Verification items for the finished model (mm, model axes). Round coordinates to 2 decimals unless told otherwise and drop trailing zeros. Order: outer loops, then holes, each group sorted by start corner. A loop starts at its lowest first (then second) coordinate and runs counter-clockwise, first axis right, second up. Notation, with made-up numbers: (80.25, 7.25) -> (119.25, 7.25) arc R28 ccw to (119.25, 45.25) -> close; hole circle Ø8 at (-28, 48). An arc over 180 degrees is marked (long way). Put each result on its own line as item: value.
Autodesk Inventor part; units mm, degrees
ref_plane "YZ Plane" through (0, 0, 0) normal (1, 0, 0) x (0, 1, 0)
ref_plane "XZ Plane" through (0, 0, 0) normal (0, 1, 0) x (-1, 0, 0)
ref_plane "XY Plane" through (0, 0, 0) normal (0, 0, 1) x (1, 0, 0)
sketch "スケッチ1" plane through (0, 0, 0) normal (0, 0, 1) x (1, 0, 0)
  line L0 (0, 0) -> (45, 0)
  line L1 (45, 0) -> (45, 100)
  line L2 (45, 100) -> (0, 100)
  line L3 (0, 100) -> (0, 0)
  dimension "d0" = 100
  dimension "d1" = 45
extrude "押し出し1" add sketch "スケッチ1" along normal blind 5
sketch "スケッチ2" plane through (0, 0, 5) normal (0, 0, 1) x (1, 0, 0)
  line L0 (0, 0) -> (45, 0)
  point P0 (22.6447, 79.5)
  dimension "d4" = 79.5
hole "穴1" at (22.6447, 79.5, 5) direction (0, 0, -1) diameter 24 end through all
sketch "スケッチ3" plane through (0, 0, 0) normal (0, 0, -1) x (-1, 0, 0)
  line L0 (0, 0) -> (-45, 0)
  line L1 (-45, 0) -> (-45, 100)
  line L2 (0, 100) -> (0, 0)
  point P0 (-10, 10)
  point P1 (-35, 10)
  dimension "d12" = 10
  dimension "d13" = 10
  dimension "d14" = 10
  dimension "d15" = 10
hole "穴2" at (10, 10, 0) at (35, 10, 0) direction (0, 0, 1) diameter 5 end through all
sketch "スケッチ4" plane through (0, 0, 5) normal (0, 0, 1) x (1, 0, 0)
  line L0 (0, 100) -> (0, 0)
  line L1 (0, 0) -> (45, 0)
  point P0 (22.5, 30)
  dimension "d23" = 22.5
  dimension "d24" = 30
hole "穴3" at (22.5, 30, 5) direction (0, 0, -1) diameter 15 depth 8 tip angle 118
properties part number "回転軸取り付け板"
Item 1: Sectioned sample at A-A, the plane y = 10. Record the boundary of the cut face in (x, z), then the cut area to 3 significant figures.
Geometry check:
outline: (0, 0) -> (7.5, 0) -> (7.5, 5) -> (0, 5) -> close; (12.5, 0) -> (32.5, 0) -> (32.5, 5) -> (12.5, 5) -> close; (37.5, 0) -> (45, 0) -> (45, 5) -> (37.5, 5) -> close
area: 175 mm2
Item 2: Release check for a two-part mould opening along Y. For faces 1 (the face through (22, 0, 2)), 2 (the face through (12.44, 9.46, 2.54)), 3 (the face through (22, 51, 0)) record: pulls with the +Y half, pulls with the -Y half, needs draft (parallel to the pull), parting line crosses it, or undercut.
Geometry check:
face 1: pulls with the -Y half
face 2: undercut
face 3: needs draft
Item 3: Sectioned sample at C-C, the plane z = 3. Record the boundary of the cut face in (x, y).
Geometry check:
outline: (0, 0) -> (45, 0) -> (45, 100) -> (0, 100) -> close; hole circle Ø5 at (10, 10); hole circle Ø24 at (22.64, 79.5); hole circle Ø15 at (22.5, 30); hole circle Ø5 at (35, 10)
Item 4: Sectioned sample at D-D, the plane y = 35. Record the boundary of the cut face in (x, z), then the cut area to 3 significant figures.
Geometry check:
outline: (0, 0) -> (16.91, 0) -> (16.91, 5) -> (0, 5) -> close; (28.09, 0) -> (45, 0) -> (45, 5) -> (28.09, 5) -> close
area: 169 mm2
Item 5: Material ranges on line 1 along Y through (x, z) = (22.5, 1.15); line 2 along X through (y, z) = (10, 3.5); line 3 along X through (y, z) = (79.5, 2.6), recorded low to high.
Geometry check:
line 1: 0 to 22.5, 37.5 to 67.5, 91.5 to 100
line 2: 0 to 7.5, 12.5 to 32.5, 37.5 to 45
line 3: 0 to 10.64, 34.64 to 45
Item 6: Sectioned sample at B-B, the plane x = 20.5. Record the boundary of the cut face in (y, z), then the cut area to 3 significant figures.
Geometry check:
outline: (0, 0) -> (22.77, 0) -> (22.77, 5) -> (0, 5) -> close; (37.23, 0) -> (67.69, 0) -> (67.69, 5) -> (37.23, 5) -> close; (91.31, 0) -> (100, 0) -> (100, 5) -> (91.31, 5) -> close
area: 310 mm2
